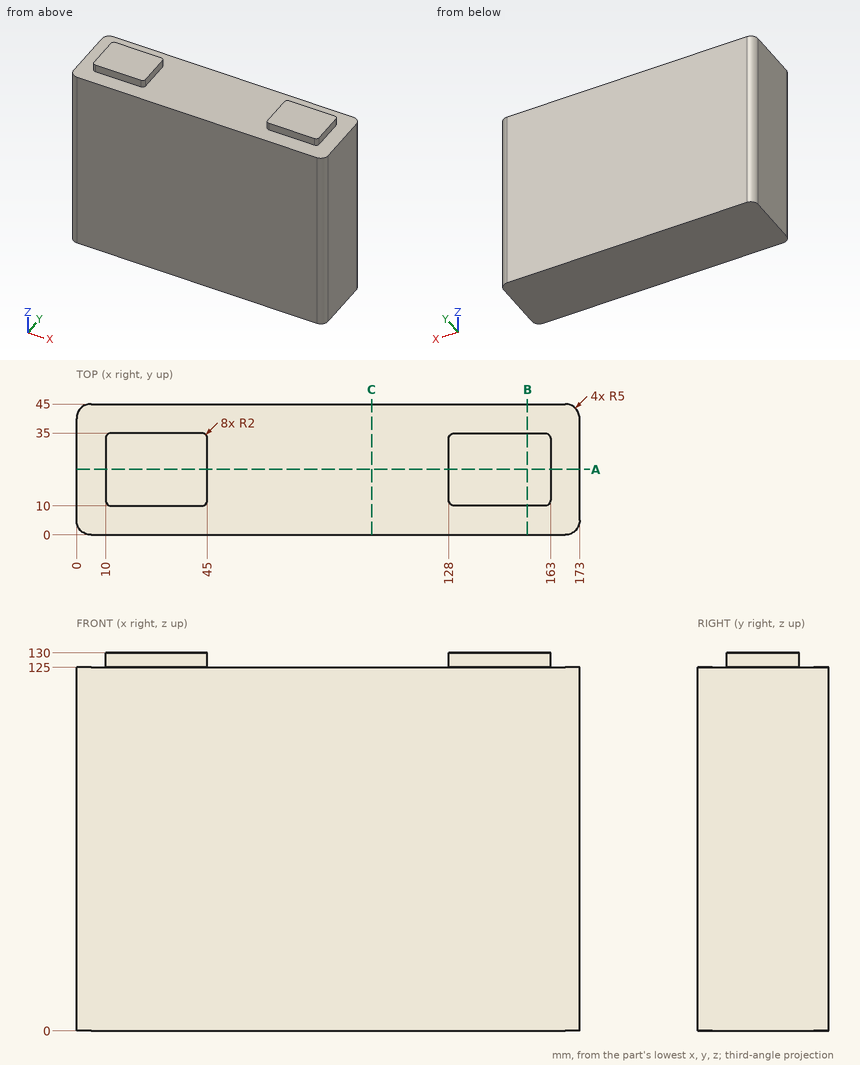
Part print with two shaded views. Sizes in mm from the minimum x, y, z corner. Round coordinates to 2 decimals unless told otherwise and drop trailing zeros. Write each loop counter-clockwise with the first axis right and the second up, starting at its lowest first coordinate (ties: lowest second). Pieces come first, ordered by that corner, then holes. Notation, with made-up numbers: M -18.75,79.5 L -6.75,79.5 A5 ccw -6.75,87.5 Z; hole C -14,4.5 d4. An arc over 180 degrees is marked long. Put each result on its own line as item: value. Start each with the question number.
1) Drill centre lines: probe 1 along Z at (x, y) = (73, 41); probe 2 along X at (y, z) = (40.5, 99.5); probe 3 along X at (y, z) = (3, 67.5). Where is each one in solid material? Low to high. Write a range as [from, to].
2) Saw through at B-B, the plane x = 155. Write the cut outline in (y, z).
3) Pin check, flat tips, straight feed: pin 1 Ø4 at (y, z) = (20, 128.5) entering from -X; pin 2 Ø2 at (y, z) = (34, 97.5) entering from -X; pin 3 Ø6 at (x, y) = (74, 12.5) entering from +Z; pin 4 Ø1.5 at (y, z) = (26.5, 128) entering from +X. Stop position of each tip, or through.
4) Saw through at C-C, the plane x = 101.5. Write the cut outline in (y, z).
5) Saw through at A-A, the plane y = 22.5. Write the cut outline in (x, z).
Resolved:
1. probe 1: [0, 125]
1. probe 2: [0.03, 172.97]
1. probe 3: [0.42, 172.58]
2. outline: M 0,0 L 45,0 L 45,125 L 35,125 L 35,130 L 10,130 L 10,125 L 0,125 Z
3. pin 1: x = 10
3. pin 2: x = 0
3. pin 3: z = 125
3. pin 4: x = 163
4. outline: M 0,0 L 45,0 L 45,125 L 0,125 Z
5. outline: M 0,0 L 173,0 L 173,125 L 163,125 L 163,130 L 128,130 L 128,125 L 45,125 L 45,130 L 10,130 L 10,125 L 0,125 Z
